Source: CAD feature listing. Evaluate the final solid. Frame: model axes, mm. Face numbers are marked on the shaded views. A direction names the side the tool comes from. Round coordinates to 2 decimals unless told otherwise and drop trailing zeros. Loops run counter-clockwise (first coordinate to the right, second up) from the corner with the lowest first, then second, coordinate; pieces in that order, holes last. Notation, with made-up numbers: (79.5, 67.5) -> (123.5, 67.5) arc R34 cw to (123.5, 97.5) -> close; hole circle Ø5 at (2, 27.5). An arc over 180 degrees is marked (long way). Return JSON: item names as keys, results as strings. Group by question number.
Autodesk Inventor part; units mm, degrees
ref_plane "YZ Plane" through (0, 0, 0) normal (1, 0, 0) x (0, 1, 0)
ref_plane "XZ Plane" through (0, 0, 0) normal (0, 1, 0) x (-1, 0, 0)
ref_plane "XY Plane" through (0, 0, 0) normal (0, 0, 1) x (1, 0, 0)
sketch "Sketch1" plane through (0, 0, 0) normal (0, 0, 1) x (1, 0, 0)
  line L0 (-64.9, 0) -> (389.4, 0)
  line L1 (0, 6.636) -> (0, -1.106)
  line L2 (0, 0) -> (0, 5.53)
  line L3 (0, 5.53) -> (3.25, 5.53)
  line L4 (3.25, 5.53) -> (3.25, 5.03)
  line L5 (3.25, 5.03) -> (5.25, 5.03)
  line L6 (5.25, 5.03) -> (5.25, 5.53)
  line L7 (5.25, 5.53) -> (22.75, 5.53)
  line L8 (22.75, 5.53) -> (22.75, 5.03)
  line L9 (22.75, 5.03) -> (37.75, 5.03)
  line L10 (37.75, 5.03) -> (37.75, 5.53)
  line L11 (37.75, 5.53) -> (320, 5.53)
  line L12 (320, 5.53) -> (320, 4)
  line L13 (320, 4) -> (324.5, 4)
  line L14 (324.5, 4) -> (324.5, 0)
  line L15 (0, 0) -> (324.5, 0)
  dimension "d0" = 37.75
  dimension "d1" = 15
  dimension "d2" = 17.5
  dimension "d3" = 2
  dimension "d4" = 11.06
  dimension "d5" = 0.5
  dimension "d6" = 0.5
  dimension "d7" = 320
  dimension "d8" = 324.5
  dimension "d9" = 8
revolve "Revolution1" add sketch "Sketch1" angle 360 about axis through (0, 0, 0) along (1, 0, 0)
chamfer "Chamfer1" distance 1.53 distance2 3 1 edges at (320, -5.53, 0) measured on face at (320, 4.9664, -0.4411)
chamfer "Chamfer2" distance 0.5 angle 45 1 edges at (324.5, -4, 0)
thread "Thread1"
equation "\"d6\" = d5"
properties part number "201-05" material "Stainless Steel"
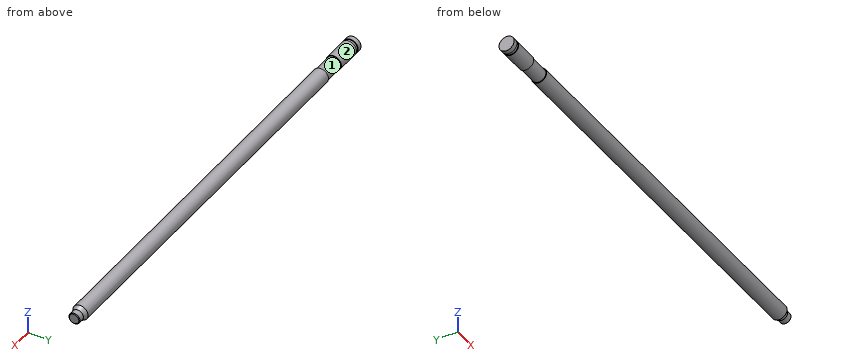
(1) Cut plane A-A (x = 47). Return loops of the section in (y, z), and give its area (3 significant figures).
(2) Set-up query: the marked faces 1 and 2. Return all of +Z, -Z, +X, -X, +Y, -Y with unobstructed straight access to the full face (end or side cutting, diameter ignored); none if empty.
(3) Pin query (flat end, axial travel): pin 1 (4 mm diameter, centred on x = 41, z = -4, fed in from -Y); pin 2 (1.5 mm diameter, centred on x = 282, y = 2.5, fed in from +Z); pin 3 (1.5 mm diameter, centred on x = 86, y = 4, fed in from -Z). Return the tip coordinate at first contact, or that it passes through.
(4) Ray query, line 1 (Y direction, x = 62, z = 2.25); line 2 (X direction, y = 5, z = -2); line 3 (X direction, y = 5.25, z = 0.5). Return the intervals inside material, ascending.
Answers follow:
{
 "1": {"outline": "circle Ø11.06 at (0, 0)", "area": "96.1 mm^2"},
 "2": {"face 1": "none", "face 2": "+X, -X"},
 "3": {"pin 1": "y = -5.16", "pin 2": "z = 5.25", "pin 3": "z = -4.47"},
 "4": {"line 1": "-5.05 to 5.05", "line 2": "0 to 3.25, 5.25 to 22.75, 37.75 to 317.28", "line 3": "0 to 3.25, 5.25 to 22.75, 37.75 to 317.5"}
}
